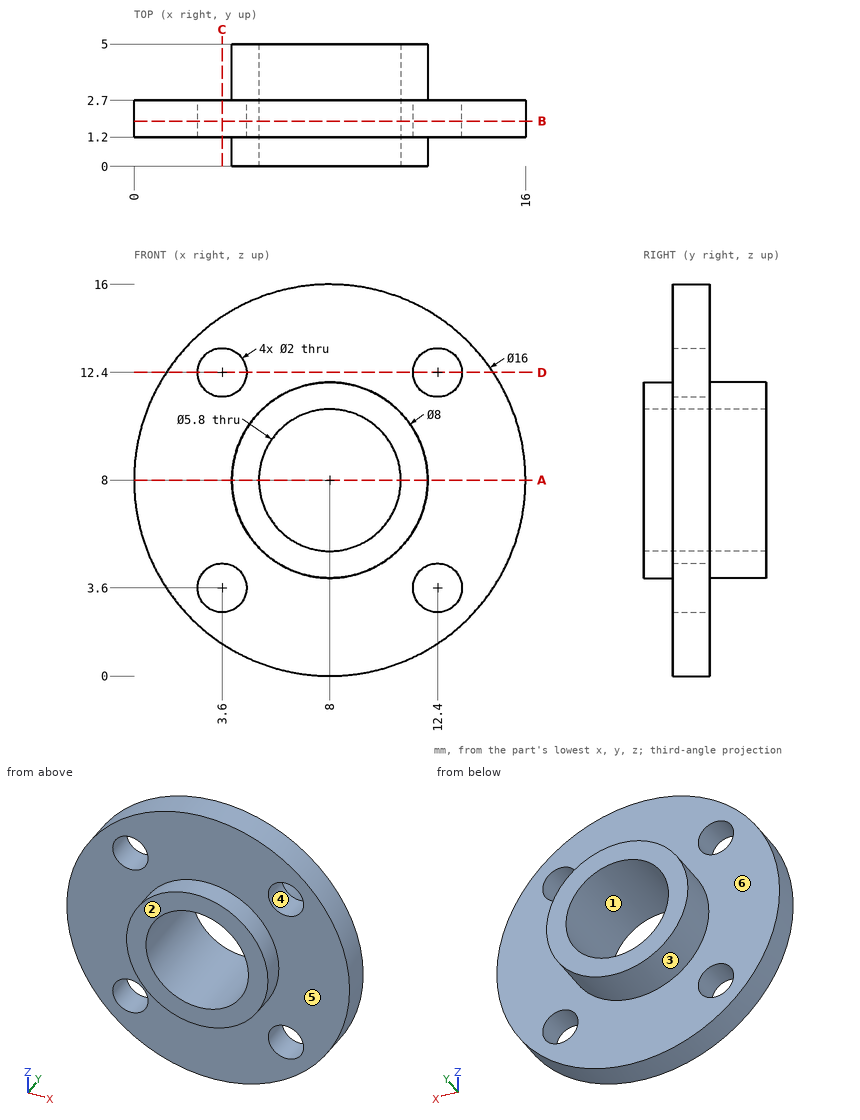
Verification items for this drawing (mm, ordinates from the low corner). A direction names the side the tool comes from. Coordinates: 2 decimals unless noted, no trailing zeros. Loops run counter-clockwise (first coordinate to the right, second up) from the corner with the lowest first, then second, coordinate; pieces in that order, holes last. Notation, with made-up numbers: (30, 33.25) - (45, 33.25) arc R6 cw to (45, 40.25) - close; hole circle Ø5 at (-35, 67.5). An arc over 180 degrees is marked (long way). Use one line per item in the form item = value. Start each with the question number.
Item 1: Mould release check, pull along X, two halves, no side actions. Record for the marked faces 1, 2 and 3: +X half, -X half, draft (parallel to the pull), parting line (faces both ways), or undercut.
Item 2: Tool access check on the marked faces 4, 5 and 6. Record the directions out of +Z, -Z, +X, -X, +Y, -Y that give a thin tool (end or side, any length) a straight path to the whole face; none if there is none.
Item 3: Section check D-D, the plane z = 12.4. Enter the section's corners in (x, y), and give its area (3 significant figures).
Item 4: Gauge pin test, flat ends, axial feed: pin 1 (1.6 mm diameter, centred on x = 3.6, z = 12.4, fed in from +Y); pin 2 (2 mm diameter, centred on x = 6.5, y = 3, fed in from -Z); pin 3 (2.5 mm diameter, centred on x = 12.4, z = 12.4, fed in from +Y); pin 4 (3 mm diameter, centred on x = 3.6, z = 3.6, fed in from -Y). Record the tip position at first contact, or that the pin passes through.
Item 5: Section check B-B, the plane y = 1.85. Enter the section's corners in (x, z), and give its area (3 significant figures).
Item 6: Section check A-A, the plane z = 8. Enter the section's corners in (x, y), and give its area (3 significant figures).
Item 7: Thickness scan on probe 1 along X at (y, z) = (2.4, 12.25); probe 2 along Z at (x, y) = (3.6, 1.9); probe 3 along Y at (x, z) = (9.5, 14.75). Record the ranges inside material, lowest first.
Item 8: Section check C-C, the plane x = 3.6. Enter the section's corners in (y, z).
Computed:
q1.face_1 = undercut
q1.face_2 = draft
q1.face_3 = parting line
q2.face_4 = +Y, -Y
q2.face_5 = -Y
q2.face_6 = +Y
q3.outline = (1.32, 1.2) - (2.6, 1.2) - (2.6, 2.7) - (1.32, 2.7) - close; (4.6, 1.2) - (11.4, 1.2) - (11.4, 2.7) - (4.6, 2.7) - close; (13.4, 1.2) - (14.68, 1.2) - (14.68, 2.7) - (13.4, 2.7) - close
q3.area = 14.0 mm2
q4.pin_1 = through
q4.pin_2 = 0.02
q4.pin_3 = 2.7
q4.pin_4 = 1.2
q5.outline = circle Ø16 at (8, 8); hole circle Ø2 at (3.6, 3.6); hole circle Ø2 at (3.6, 12.4); hole circle Ø5.8 at (8, 8); hole circle Ø2 at (12.4, 3.6); hole circle Ø2 at (12.4, 12.4)
q5.area = 162 mm2
q6.outline = (0, 1.2) - (4, 1.2) - (4, 0) - (5.1, 0) - (5.1, 5) - (4, 5) - (4, 2.7) - (0, 2.7) - close; (10.9, 0) - (12, 0) - (12, 1.2) - (16, 1.2) - (16, 2.7) - (12, 2.7) - (12, 5) - (10.9, 5) - close
q6.area = 23.0 mm2
q7.probe_1 = 1.22 to 2.61, 4.59 to 11.41, 13.39 to 14.78
q7.probe_2 = 1.32 to 2.6, 4.6 to 11.4, 13.4 to 14.68
q7.probe_3 = 1.2 to 2.7
q8.outline = (1.2, 1.32) - (2.7, 1.32) - (2.7, 2.6) - (1.2, 2.6) - close; (1.2, 4.6) - (2.7, 4.6) - (2.7, 11.4) - (1.2, 11.4) - close; (1.2, 13.4) - (2.7, 13.4) - (2.7, 14.68) - (1.2, 14.68) - close
